CAD build for the part. Positions are in the model's coordinates, mm. A direction names the side the tool comes from. Coordinates: 2 decimals unless noted, no trailing zeros. Loops run counter-clockwise (first coordinate to the right, second up) from the corner with the lowest first, then second, coordinate; pieces in that order, holes last.
1) Saw through at C-C, the plane y = -4.5. Write the cut outline in (x, z), and give its area (3 significant figures).
2) Two-plate mould, pull along Z, no slides. Class faces 3 (the flat face through (-98, -1.2, 17)), 4 (the flat face through (-107.4, -35.6, 25)), 5 (the flat face through (-64, -35, 0)), 6 (the flat face through (-108, -35, 8)): +Z half, -Z half, draft (parallel to the pull), parting line (faces both ways), or undercut.
3) Saw through at D-D, the plane x = -28.5. Write the cut outline in (y, z), and give its area (3 significant figures).
4) Pin check, flat tips, straight feed: pin 1 Ø13 at (x, y) = (-106.5, -23) entering from -Z; pin 2 Ø1 at (x, z) = (-72, 12) entering from -Y; pin 3 Ø1.3 at (x, y) = (-81.5, -5.5) entering from -Z; pin 4 Ø1 at (x, z) = (-115, 20) entering from -Y. Stop position of each tip, or through.
5) Saw through at B-B, the plane x = -100. Write the cut outline in (y, z), and give its area (3 significant figures).
6) Saw through at A-A, the plane y = -21. Write the cut outline in (x, z).
7) Wall check: line 1 along X through (y, z) = (-9.5, 24); line 2 along X through (y, z) = (-6, 10); line 3 along X through (y, z) = (-13.5, 14). Give the ranges that are in metal, low to high.
8) Which spindle directions (+Z, -Z, +X, -X, +Y, -Y) get a long thin tool onto all of the face, cutting with end or side? Do faces 1 (the flat face through (-30, -1.2, 17)), 2 (the flat face through (4.822, -18, 17)). Say none if no direction does.
```python
from build123d import *

# Parameters (mm, degrees)
F0_W      = 120
F0_H      = 36
F1_DEPTH  = 35
F2_W      = 7
F2_H      = 20
F3_DEPTH  = 1.2
F4_W      = 11.6417678248
F4_H      = 18
F5_DEPTH  = 1.201
F6_W      = 25
F6_H      = 17
F7_DEPTH  = 1.2
F8_W      = 1.2
F8_H      = 17
F9_DEPTH  = 3
F10_W     = 25
F10_H     = 17
F11_DEPTH = 1.2


with BuildPart() as f1:
    # F0 (on Top) → F1 (new body)
    with BuildSketch(Plane.XY):
        with Locations((-55.1781901717, -18)):
            Rectangle(F0_W, F0_H)
        Polygon((-113.9781901717, -34.8), (-113.9781901717, -1.2), (-107.9781901717, -1.2), (-89.9781901717, -1.2), (-82.1781901717, -1.2), (-80.9781901717, -1.2), (-63.9781901717, -1.2), (-62.7781901717, -1.2), (-49.0207746625, -1.2), (-45.235440135, -1.2), (3.6218098283, -1.2), (3.6218098283, -34.8), (-62.7781901717, -34.8), (-63.9781901717, -34.8), (-80.9781901717, -34.8), (-82.1781901717, -34.8), align=None, mode=Mode.SUBTRACT)
        Polygon((-82.1781901717, -26.7), (-82.1781901717, -34.8), (-80.9781901717, -34.8), (-80.9781901717, -26.6408454627), (-80.9781901717, -8.1258974969), (-80.9781901717, -1.2), (-82.1781901717, -1.2), (-82.1781901717, -8.7), align=None)
        Polygon((-63.9781901717, -26.6408454627), (-63.9781901717, -34.8), (-62.7781901717, -34.8), (-62.7781901717, -1.2), (-63.9781901717, -1.2), (-63.9781901717, -8.1258974969), align=None)
    extrude(amount=F1_DEPTH)

    # F2 (on face) → F3 (cut)
    with BuildSketch(Plane.YZ.offset(-80.9781901717)):
        with Locations((-5.5, 10)):
            Rectangle(F2_W, F2_H)
    extrude(amount=-F3_DEPTH, mode=Mode.SUBTRACT)

    # F4 (on face) → F5 (cut, through all)
    with BuildSketch(Plane(origin=(0, -34.8, 0), x_dir=(-1, 0, 0), z_dir=(0, 1, 0))):
        with Locations((72.271104902, 17)):
            Rectangle(F4_W, F4_H)
    extrude(amount=-F5_DEPTH, mode=Mode.SUBTRACT)

    # F6 (on face) → F7 (cut)
    with BuildSketch(Plane(origin=(0, -34.8, 0), x_dir=(-1, 0, 0), z_dir=(0, 1, 0))):
        with Locations((100.0405803323, 16.5)):
            Rectangle(F6_W, F6_H)
    extrude(amount=-F7_DEPTH, mode=Mode.SUBTRACT)

    # F8 (on face) → F9 (cut)
    with BuildSketch(Plane.YZ.offset(-112.5405803323)):
        with Locations((-35.4, 16.5)):
            Rectangle(F8_W, F8_H)
    extrude(amount=-F9_DEPTH, mode=Mode.SUBTRACT)

    # F10 (on face) → F11 (cut)
    with BuildSketch(Plane(origin=(-115.1781901717, 0, 0), x_dir=(0, -1, 0), z_dir=(-1, 0, 0))):
        with Locations((22.3, 16.5)):
            Rectangle(F10_W, F10_H)
    extrude(amount=-F11_DEPTH, mode=Mode.SUBTRACT)


solid = f1.part
```
Data:
1. outline: (-115.18, 0) - (-113.98, 0) - (-113.98, 35) - (-115.18, 35) - close; (-82.18, 20) - (-80.98, 20) - (-80.98, 35) - (-82.18, 35) - close; (-63.98, 0) - (-62.78, 0) - (-62.78, 35) - (-63.98, 35) - close; (3.62, 0) - (4.82, 0) - (4.82, 35) - (3.62, 35) - close
1. area: 144 mm2
2. face 3: draft
2. face 4: undercut
2. face 5: -Z half
2. face 6: undercut
3. outline: (-36, 0) - (-34.8, 0) - (-34.8, 35) - (-36, 35) - close; (-1.2, 0) - (0, 0) - (0, 35) - (-1.2, 35) - close
3. area: 84.0 mm2
4. pin 1: passes through
4. pin 2: stops at y = -1.2
4. pin 3: stops at z = 20
4. pin 4: stops at y = -9.8
5. outline: (-36, 0) - (-34.8, 0) - (-34.8, 8) - (-36, 8) - close; (-36, 25) - (-34.8, 25) - (-34.8, 35) - (-36, 35) - close; (-1.2, 0) - (0, 0) - (0, 35) - (-1.2, 35) - close
5. area: 63.6 mm2
6. outline: (-115.18, 0) - (-113.98, 0) - (-113.98, 8) - (-115.18, 8) - close; (-115.18, 25) - (-113.98, 25) - (-113.98, 35) - (-115.18, 35) - close; (-82.18, 0) - (-80.98, 0) - (-80.98, 35) - (-82.18, 35) - close; (-63.98, 0) - (-62.78, 0) - (-62.78, 35) - (-63.98, 35) - close; (3.62, 0) - (4.82, 0) - (4.82, 35) - (3.62, 35) - close
7. line 1: x = -115.18 to -113.98, -82.18 to -80.98, -63.98 to -62.78, 3.62 to 4.82
7. line 2: x = -115.18 to -113.98, -63.98 to -62.78, 3.62 to 4.82
7. line 3: x = -82.18 to -80.98, -63.98 to -62.78, 3.62 to 4.82
8. face 1: +Z, -Z
8. face 2: +Z, -Z, +X, +Y, -Y
